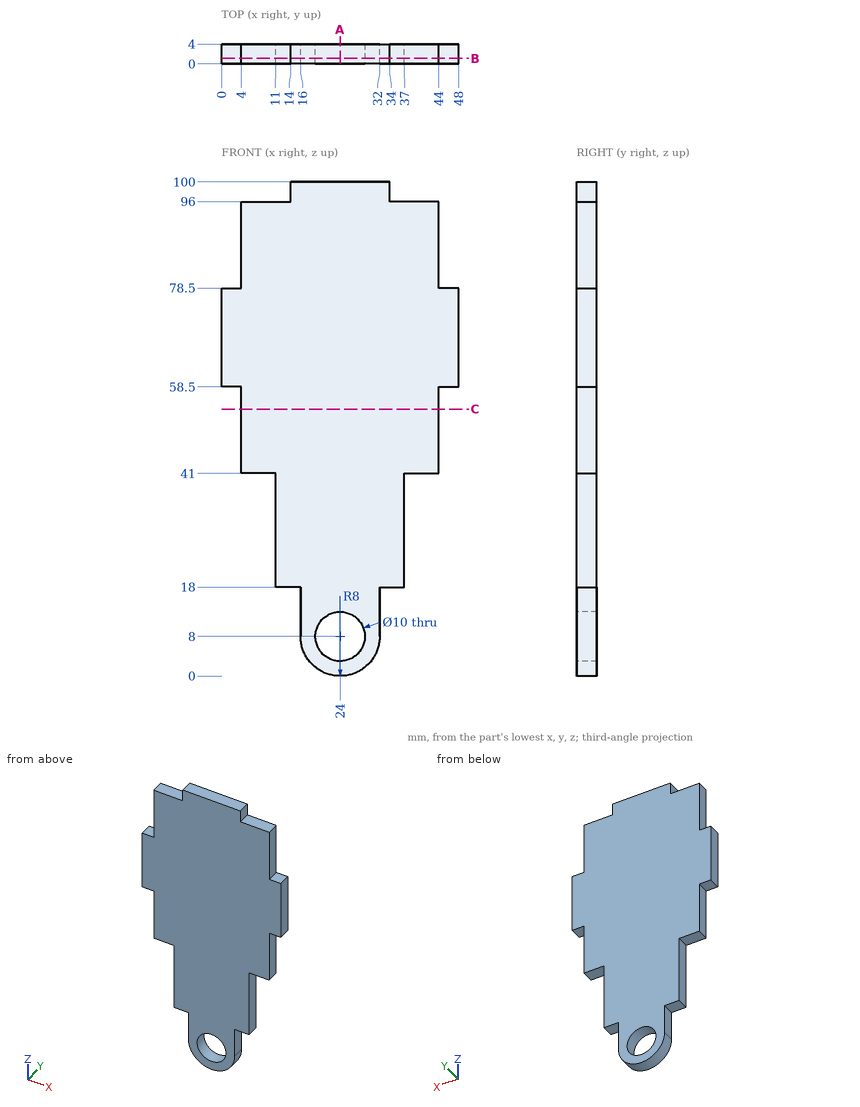
Answer from the drawing. Dimensions are ordinates in mm from the lowest x, y and z of the part. Coordinates: 2 decimals unless noted, no trailing zeros. Loops run counter-clockwise (first coordinate to the right, second up) from the corner with the lowest first, then second, coordinate; pieces in that order, holes last.
1) Section C-C (z = 54) is taken. Give the vertices of the cut face in (x, y), plus the area to 3 significant figures.
Results:
outline: (4, 0) - (44, 0) - (44, 4) - (4, 4) - close
area: 160 mm2
2) Flat-ended cylindrical pins translate along their axes: pin 1 (1.2 mm diameter, centred on y = 1.5, z = 84.5, fed in from -X); pin 2 (2 mm diameter, centred on y = 2, z = 34, fed in from +X); pin 3 (2 mm diameter, centred on y = 2, z = 87.5, fed in from +X). Find the tip coordinate at first contact, or state that the pin passes through.
Results:
pin 1: stops at x = 4
pin 2: stops at x = 37
pin 3: stops at x = 44
3) Section A-A (x = 24) is taken. Give the vertices of the cut face in (y, z), plus the area to 3 significant figures.
Results:
outline: (0, 0) - (4, 0) - (4, 3) - (0, 3) - close; (0, 13) - (4, 13) - (4, 100) - (0, 100) - close
area: 360 mm2
4) Consider probe 1 along Z at (x, y) = (24, 2.5); probe 2 along X at (y, z) = (2.7, 34); probe 3 along X at (y, z) = (0.9, 82.5). Determine where each line is inside the solid, lowest interval first.
Results:
probe 1: z = 0 to 3, 13 to 100
probe 2: x = 11 to 37
probe 3: x = 4 to 44
5) Section B-B (y = 1.1) is taken. Give the vertices of the cut face in (x, z), plus the area to 3 significant figures.
Results:
outline: (0, 58.5) - (4, 58.5) - (4, 41) - (11, 41) - (11, 18) - (16, 18) - (16, 8) arc R8 ccw to (32, 8) - (32, 18) - (37, 18) - (37, 41) - (44, 41) - (44, 58.5) - (48, 58.5) - (48, 78.5) - (44, 78.5) - (44, 96) - (34, 96) - (34, 100) - (14, 100) - (14, 96) - (4, 96) - (4, 78.5) - (0, 78.5) - close; hole circle Ø10 at (24, 8)
area: 3,220 mm2
